from build123d import *

# Parameters (mm, degrees)
F0_W     = 558.8
F0_H     = 457.2
F1_DEPTH = 19.05
F3_D     = 5.1054


with BuildPart() as f1:
    # F0 (on Top) → F1 (new body)
    with BuildSketch(Plane.XY):
        with Locations((29.861329, -21.937743)):
            Rectangle(F0_W, F0_H)
    extrude(amount=F1_DEPTH)

    # F3 (through all)
    with Locations(Plane.XY.offset(19.05)):
        with Locations((-236.838671, -34.637743), (-236.838671, 66.962257), (144.161329, 193.962257), (-186.038671, 193.962257), (296.561329, -161.637743), (-33.638671, 193.962257), (93.361329, -237.837743), (118.761329, 193.962257), (245.761329, -237.837743), (220.361329, 193.962257), (93.361329, 193.962257), (296.561329, -110.837743), (296.561329, 117.762257), (271.161329, 193.962257), (-84.438671, -237.837743), (296.561329, -237.837743), (296.561329, -9.237743), (-211.438671, -237.837743), (17.161329, -237.837743), (-160.638671, -237.837743), (296.561329, 143.162257), (-135.238671, 193.962257), (194.961329, 193.962257), (296.561329, -34.637743), (-236.838671, -85.437743), (296.561329, 66.962257), (-135.238671, -237.837743), (-236.838671, 117.762257), (17.161329, 193.962257), (-236.838671, -187.037743), (-236.838671, 143.162257), (-236.838671, 41.562257), (-236.838671, 16.162257), (296.561329, -85.437743), (42.561329, 193.962257), (-59.038671, -237.837743), (-236.838671, 92.362257), (-59.038671, 193.962257), (271.161329, -237.837743), (-109.838671, 193.962257), (-236.838671, -161.637743), (67.961329, -237.837743), (296.561329, -60.037743), (-160.638671, 193.962257), (169.561329, -237.837743), (-236.838671, -136.237743), (-236.838671, -212.437743), (-186.038671, -237.837743), (-8.238671, -237.837743), (-236.838671, -110.837743), (118.761329, -237.837743), (-236.838671, -237.837743), (-33.638671, -237.837743), (296.561329, -136.237743), (296.561329, 41.562257), (-236.838671, 168.562257), (-211.438671, 193.962257), (-236.838671, 193.962257), (169.561329, 193.962257), (296.561329, -212.437743), (220.361329, -237.837743), (-236.838671, -60.037743), (-109.838671, -237.837743), (321.961329, 193.962257), (-84.438671, 193.962257), (-236.838671, -9.237743), (245.761329, 193.962257), (296.561329, -187.037743), (296.561329, 193.962257), (-8.238671, 193.962257), (144.161329, -237.837743), (194.961329, -237.837743), (296.561329, 168.562257), (42.561329, -237.837743), (67.961329, 193.962257), (296.561329, 92.362257), (296.561329, 16.162257)):
            Hole(F3_D / 2)


solid = f1.part
Design review of the part built by this model. Coordinates are the model's own, in mm. Coordinates: 2 decimals unless noted, no trailing zeros. Use one line per item in the form item = value.
Q1. Insertion check: pin 1 Ø4 at (x, y) = (42.56, -237.84) entering from +Z. The pin has a flat end and moves straight along its axis. Give the tip position at first contact, or say it passes through.
Taken from the geometry:
pin_1 = through
Q2. The part is to be moulded in two halves that separate along Z. For faces 1 (the flat face through (26, -19, 19.05)), 2 (the flat face through (26, 206.662, 9)), 3 (the flat face through (26, -19, 0)), say which applies: +Z half, -Z half, draft (parallel to the pull), parting line (faces both ways), or undercut.
Taken from the geometry:
face_1 = +Z half
face_2 = draft
face_3 = -Z half
Q3. For probe 1 along X at (y, z) = (117, 12.5); probe 2 along Y at (x, z) = (-107.5, 14.25); probe 3 along X at (y, z) = (-163, 16.5), list the stretches that pass through material, from the lowest coordinate up.
Taken from the geometry:
probe_1 = -249.54 to -239.27, -234.4 to 294.13, 299 to 309.26
probe_2 = -250.54 to -238.86, -236.81 to 192.94, 194.99 to 206.66
probe_3 = -249.54 to -239, -234.68 to 294.4, 298.72 to 309.26
